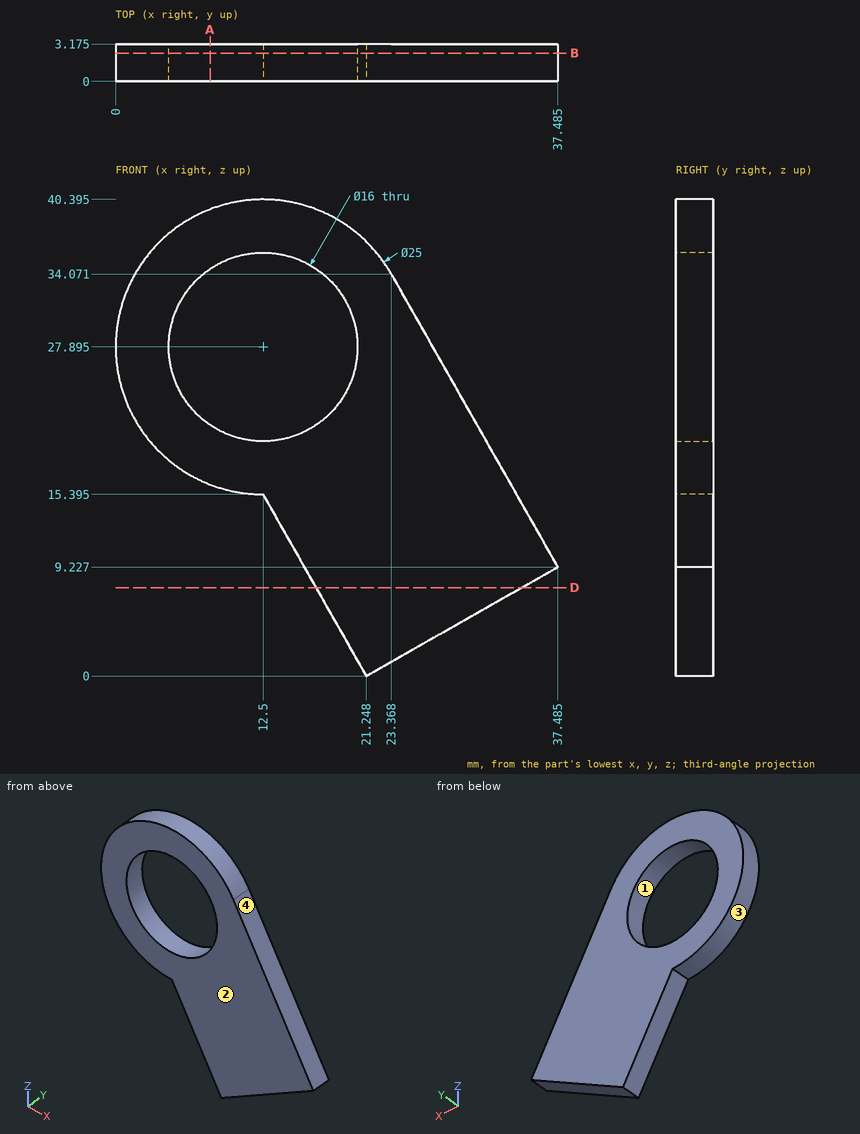
Could you check a few things on this drawing? It's one solid part, dimensions in mm from its lowest x, y, z. Coordinates: 2 decimals unless noted, no trailing zeros. Loops run counter-clockwise (first coordinate to the right, second up) from the corner with the lowest first, then second, coordinate; pieces in that order, holes last.
1. We'd pull the mould along X, two halves only. Please class the marked faces 1, 2, 3 and 4: released by +X, released by -X, zero draft, split by the parting line, or undercut.
2. Imagine slicing it at A-A (x = 8). Please give me the cut outline in (y, z) (1 decimal).
3. Imagine slicing it at B-B (y = 2.4). Please give me the cut outline in (x, z) (1 decimal), and give its area (3 significant figures).
4. Imagine slicing it at D-D (z = 7.5). Please give me the cut outline in (x, y) (1 decimal).
5. For P1, Ø18.5, axis at x = 12.5, z = 27.9, coming from the +Y side (3 decimals), with a flat end and sliding along its axis, tell me the tip position at first contact or that it passes through.
6. I need wall thicknesses on L1, parallel to Z at x = 13.5, y = 1.8 (1 decimal); L2, parallel to X at y = 1.5, z = 31; L3, parallel to X at y = 1.1, z = 31.5. Which ranges of each line are inside material? Lowest first, please.
Computed values:
1. face 1: undercut
1. face 2: zero draft
1. face 3: split by the parting line
1. face 4: released by +X
2. outline: (0, 16.2) - (3.2, 16.2) - (3.2, 21.3) - (0, 21.3) - close; (0, 34.5) - (3.2, 34.5) - (3.2, 39.6) - (0, 39.6) - close
3. outline: (12.5, 15.4) - (21.2, 0) - (37.5, 9.2) - (23.4, 34.1) arc R12.5 ccw (long way) to start; hole circle Ø16 at (12.5, 27.9)
3. area: 627 mm2
4. outline: (17, 0) - (34.4, 0) - (34.4, 3.2) - (17, 3.2) - close
5. P1: stops at y = 3.175
6. L1: z = 13.6 to 20, 35.8 to 40.4
6. L2: x = 0.39 to 5.13, 19.87 to 25.11
6. L3: x = 0.53 to 5.36, 19.64 to 24.83
